from build123d import *

# Parameters (mm, degrees)
SALIENTE_EXTRUIR1_DEPTH = 9
CROQUIS2_R              = 3.5
CORTAR_EXTRUIR1_DEPTH   = 10
CROQUIS3_R              = 1.5
CORTAR_EXTRUIR2_DEPTH   = 10


with BuildPart() as part:
    # Croquis1 → Saliente-Extruir1 (new body)
    with BuildSketch(Plane(origin=(0, 0, 0), x_dir=(1, 0, 0), z_dir=(0, 1, 0))):
        Polygon((0, 2.473088065), (2.473088065, 0), (32.526911935, 0), (35, 2.473088065), (35, 32.526911935), (32.526911935, 35), (2.473088065, 35), (0, 32.526911935), align=None)
    extrude(amount=SALIENTE_EXTRUIR1_DEPTH)

    # Croquis2 → Cortar-Extruir1 (cut, through all)
    with BuildSketch(Plane(origin=(0, 9, 0), x_dir=(1, 0, 0), z_dir=(0, 1, 0))):
        with Locations((17.5, 17.5)):
            Circle(CROQUIS2_R)
    extrude(amount=-CORTAR_EXTRUIR1_DEPTH, mode=Mode.SUBTRACT)

    # Croquis3 → Cortar-Extruir2 (cut, through all)
    with BuildSketch(Plane(origin=(0, 9, 0), x_dir=(1, 0, 0), z_dir=(0, 1, 0))):
        with Locations((4.5, 30.5)):
            Circle(CROQUIS3_R)
        with Locations((30.5, 30.5)):
            Circle(CROQUIS3_R)
        with Locations((30.5, 4.5)):
            Circle(CROQUIS3_R)
        with Locations((4.5, 4.5)):
            Circle(CROQUIS3_R)
    extrude(amount=-CORTAR_EXTRUIR2_DEPTH, mode=Mode.SUBTRACT)


solid = part.part
Source: CAD feature listing. Evaluate the final solid. Frame: model axes, mm. Give positions to 0.01 mm unless a question says otherwise; leave off trailing zeros. Write each loop counter-clockwise with the first axis right and the second up, starting at its lowest first coordinate (ties: lowest second). Pieces come first, ordered by that corner, then holes. Notation, with made-up numbers: M -14.5,72 L 10.5,72 A17 ccw 10.5,91 Z; hole C 2.25,-8.5 d8. An arc over 180 degrees is marked long. Answer as a JSON object with one key per item and string values.
Q1. Cut plane A-A, the plane x = 17.5. Return the cut outline in (y, z), then the cut area to 3 significant figures.
Geometry check:
{"outline": "M 0,-35 L 9,-35 L 9,-21 L 0,-21 Z; M 0,-14 L 9,-14 L 9,0 L 0,0 Z", "area": "252 mm^2"}
Q2. Ray query, line 1 along Z through (x, y) = (30.5, 6.5); line 2 along X through (y, z) = (4, -30.5); line 3 along Z through (x, y) = (5, 6). Return the intervals inside material, ascending.
Geometry check:
{"line 1": "z = -35 to -32, -29 to -6, -3 to 0", "line 2": "x = 0 to 3, 6 to 29, 32 to 35", "line 3": "z = -35 to -31.91, -29.09 to -5.91, -3.09 to 0"}
Q3. Cut plane D-D, the plane z = -17.5. Return the cut outline in (x, y), then the cut area to 3 significant figures.
Geometry check:
{"outline": "M 0,0 L 14,0 L 14,9 L 0,9 Z; M 21,0 L 35,0 L 35,9 L 21,9 Z", "area": "252 mm^2"}
Q4. Cut plane C-C, the plane y = 2. Return the cut outline in (x, z), then the cut area to 3 significant figures.
Geometry check:
{"outline": "M 0,-32.53 L 2.47,-35 L 32.53,-35 L 35,-32.53 L 35,-2.47 L 32.53,0 L 2.47,0 L 0,-2.47 Z; hole C 4.5,-30.5 d3; hole C 4.5,-4.5 d3; hole C 17.5,-17.5 d7; hole C 30.5,-30.5 d3; hole C 30.5,-4.5 d3", "area": "1,150 mm^2"}
Q5. Cut plane B-B, the plane z = -30.5. Return the cut outline in (x, y), then the cut area to 3 significant figures.
Geometry check:
{"outline": "M 0,0 L 3,0 L 3,9 L 0,9 Z; M 6,0 L 29,0 L 29,9 L 6,9 Z; M 32,0 L 35,0 L 35,9 L 32,9 Z", "area": "261 mm^2"}
